CAD build for the part. Positions are in the model's coordinates, mm. Face numbers are marked on the shaded views. A direction names the side the tool comes from. Give positions to 0.01 mm unless a question says otherwise; leave off trailing zeros. Write each loop counter-clockwise with the first axis right and the second up, starting at its lowest first coordinate (ties: lowest second). Pieces come first, ordered by that corner, then holes. Notation, with made-up numbers: (-34.5, 64.5) - (-2.5, 64.5) arc R15 cw to (-2.5, 72.5) - close; hole circle Ø5 at (51, -9). An arc over 180 degrees is marked (long way). Put each result on its own line as item: value. Start each with the question number.
1. Cut at C-C on z = 15.2. List the corners of the cut face in (x, y), and give its area (3 significant figures).
2. Wall check: line 1 (Y direction, x = 25.75, z = 15.2); line 2 (Y direction, x = 28.5, z = 8.25); line 3 (X direction, y = 12, z = 8.4). Give the ranges that are in metal, low to high.
3. Tool access for the marked faces 1, 2 and 3: list every direction of +Z, -Z, +X, -X, +Y, -Y with a clear straight run to the whole face (end or side of a thin tool).
4. Mould opens along Y. For the marked faces 4, 5 and 6 say: +Y half, -Y half, draft (parallel to the pull), parting line (faces both ways), or undercut.
5. Cut at A-A on y = 20.5. List the corners of the cut face in (x, z).
6. Drop flat-ended pins along their axis: pin 1 (4 mm diameter, centred on x = 26, y = 2, fed in from -Z); pin 2 (2.5 mm diameter, centred on x = 25.5, y = 2.5, fed in from +Z). Give the stop position or say it passes through.
7. Cut at D-D on y = 12. List the corners of the cut face in (x, z), and give its area (3 significant figures).
8. Cut at B-B on x = 26. Give the number of separate pieces and of enclosed holes in the cut face, and give its area (3 significant figures).
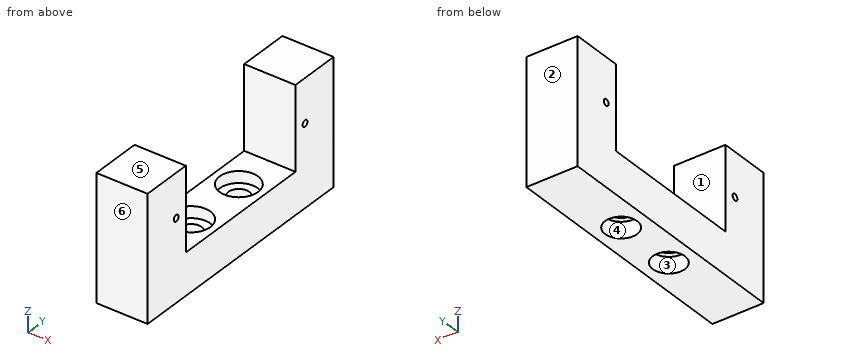
from build123d import *

# Parameters (mm, degrees)
PAD003_DEPTH            = 8
HOLE_D                  = 3.3
HOLE_DEPTH              = 25
HOLE_CBORE_D            = 6
HOLE_CBORE_DEPTH        = 1.8
SKETCH010_R             = 0.5
POCKET004_DEPTH         = 8.001
SKETCH008_R             = 2.5
POCKET005_DEPTH         = 2.5
BODY003_PITCH_ANGLE     = 90
BODY003_PLACEMENT_ANGLE = -180


with BuildPart() as part:
    # Sketch009 → Pad003 (new body)
    with BuildSketch(Plane.XY):
        Polygon((0, 19.5), (0, 11.5), (13, 11.5), (13, -11.5), (0, -11.5), (0, -19.5), (19.5, -19.5), (19.5, 19.5), align=None)
    extrude(amount=PAD003_DEPTH)

    # Hole
    with Locations(Plane(origin=(13, 0, 0), x_dir=(0, -1, 0), z_dir=(-1, 0, 0))):
        with Locations((-5, 4), (5, 4)):
            CounterBoreHole(HOLE_D / 2, HOLE_CBORE_D / 2, HOLE_CBORE_DEPTH, depth=HOLE_DEPTH)

    # Sketch010 (on Face5 of Hole) → Pocket004 (cut, through all)
    with BuildSketch(Plane.XY.offset(8)):
        with Locations((6.8, 13.5)):
            Circle(SKETCH010_R)
        with Locations((6.8, -13.5)):
            Circle(SKETCH010_R)
    extrude(amount=-POCKET004_DEPTH, mode=Mode.SUBTRACT)

    # Sketch008 (on Face6 of Pocket004) → Pocket005 (cut)
    with BuildSketch(Plane.YZ.offset(19.5)):
        with Locations((-5, 4)):
            Circle(SKETCH008_R)
        with Locations((5, 4)):
            Circle(SKETCH008_R)
    extrude(amount=-POCKET005_DEPTH, mode=Mode.SUBTRACT)


with BuildPart() as part_1:
    # Body003 pitch: moved
    add(part.part.rotate(Axis((0, 0, 0), (0, 1, 0)), BODY003_PITCH_ANGLE))


with BuildPart() as part_2:
    # Body003 placement: moved
    add(part_1.part.moved(Location((30, 7, 22))).rotate(Axis((30, 7, 22), (0, 0, 1)), BODY003_PLACEMENT_ANGLE))


solid = part_2.part
Report:
1. outline: (22, -12.5) - (30, -12.5) - (30, -7) - (22, -7) - close; (22, -6) - (30, -6) - (30, -4.5) - (22, -4.5) - close; (22, 18.5) - (30, 18.5) - (30, 20) - (22, 20) - close; (22, 21) - (30, 21) - (30, 26.5) - (22, 26.5) - close
1. area: 112 mm²
2. line 1: y = -12.5 to -7, -6 to -4.5, 18.5 to 20, 21 to 26.5
2. line 2: y = -12.5 to 0.34, 3.66 to 10.34, 13.66 to 26.5
2. line 3: x = 22 to 23, 29 to 30
3. face 1: +Z, +X, -X
3. face 2: +Z, -Z, +X, -X, +Y
3. face 3: -Z
4. face 4: undercut
4. face 5: draft
4. face 6: -Y half
5. outline: (22, 2.5) - (30, 2.5) - (30, 14.7) - (22, 14.7) - close; (22, 15.7) - (30, 15.7) - (30, 22) - (22, 22) - close
6. pin 1: stops at z = 5
6. pin 2: stops at z = 7.2
7. outline: (22, 2.5) - (23.5, 2.5) - (23.5, 5) - (24.35, 5) - (24.35, 7.2) - (23, 7.2) - (23, 9) - (22, 9) - close; (27.65, 5) - (28.5, 5) - (28.5, 2.5) - (30, 2.5) - (30, 9) - (29, 9) - (29, 7.2) - (27.65, 7.2) - close
7. area: 21.4 mm²
8. separate pieces: 3
8. enclosed holes: 2
8. area: 399 mm²
